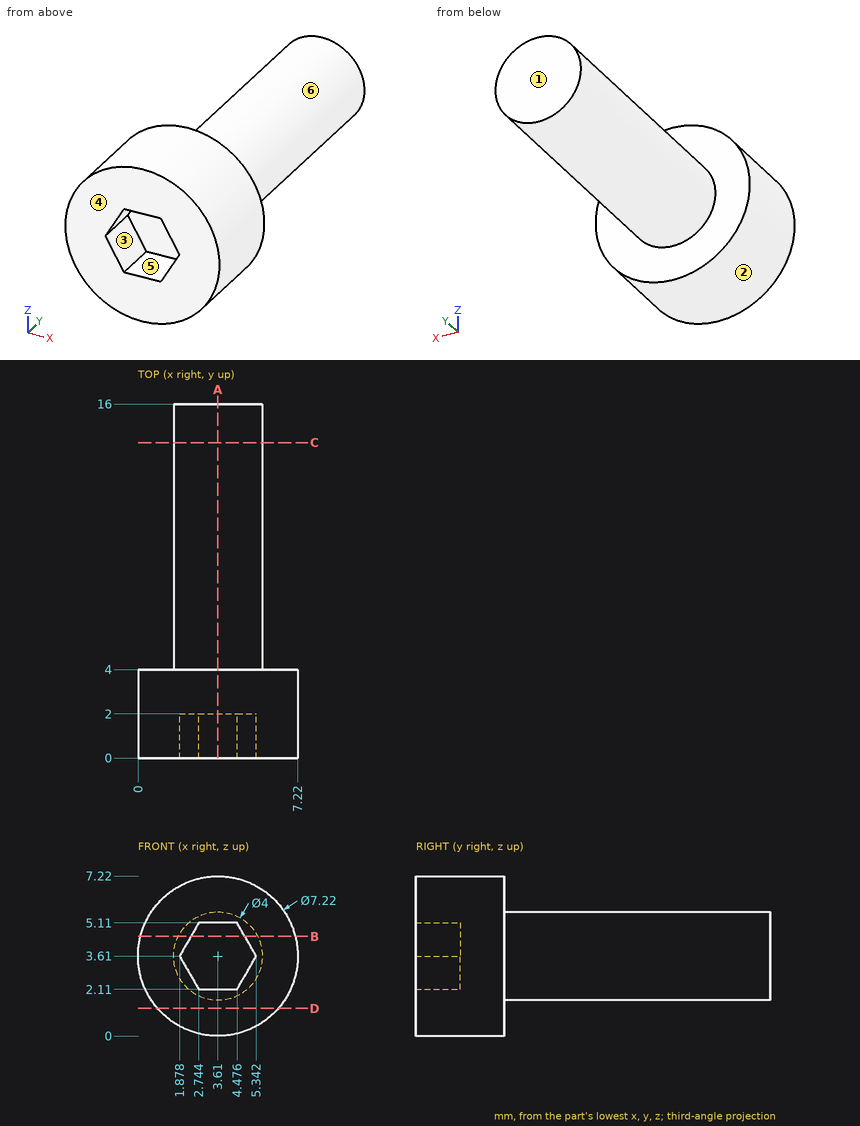
Source: three-view drawing plus pictorial views. Frame: mm from the lowest corner of the part. A direction names the side the tool comes from. Coordinates: 2 decimals unless noted, no trailing zeros. Order: outer loops, then holes, each group sorted by start corner. A loop starts at its lowest first (then second) coordinate and runs counter-clockwise, first axis right, second up. Notation, with made-up numbers: M 27.25,50 L 35.25,50 A30 ccw 35.25,83 Z; hole C 1.5,53.5 d10. An arc over 180 degrees is marked long. Answer in a Markdown table with one row per item.
(1) Section query B-B, the plane z = 4.5. Output: boundary loops of the cut face in (x, y), plus the area to 3 significant figures.
Numbers:
| item | result |
|---|---|
| outline | M 0.11,0 L 2.39,0 L 2.39,2 L 4.83,2 L 4.83,0 L 7.11,0 L 7.11,4 L 5.4,4 L 5.4,16 L 1.82,16 L 1.82,4 L 0.11,4 Z |
| area | 66.1 mm^2 |
(2) Draft query along X for the marked faces 1, 2 and 3. Return one class per face: pulls with the +X half, pulls with the -X half, needs draft (parallel to the pull), parting line crosses it, or undercut.
Numbers:
| item | result |
|---|---|
| face 1 | needs draft |
| face 2 | parting line crosses it |
| face 3 | undercut |
(3) Section query D-D, the plane z = 1.25. Output: boundary loops of the cut face in (x, y).
Numbers:
| item | result |
|---|---|
| outline | M 0.88,0 L 6.34,0 L 6.34,4 L 0.88,4 Z |
(4) Material intervals for line 1 (Y direction, x = 4.5, z = 0.5); line 2 (Y direction, x = 4.5, z = 3.25); line 3 (Z direction, x = 3.5, y = 5), sorted ascending. Write a range as [from, to].
Numbers:
| item | result |
|---|---|
| line 1 | y = [0, 4] |
| line 2 | y = [2, 16] |
| line 3 | z = [1.61, 5.61] |
(5) Section query A-A, the plane x = 3.61. Output: boundary loops of the cut face in (y, z).
Numbers:
| item | result |
|---|---|
| outline | M 0,0 L 4,0 L 4,1.61 L 16,1.61 L 16,5.61 L 4,5.61 L 4,7.22 L 0,7.22 L 0,5.11 L 2,5.11 L 2,2.11 L 0,2.11 Z |
(6) Section query C-C, the plane y = 14.25. Output: boundary loops of the cut face in (x, z).
Numbers:
| item | result |
|---|---|
| outline | C 3.61,3.61 d4 |
(7) Access query for the marked faces 4, 5 and 6. Directions: +Z, -Z, +X, -X, +Y, -Y. A direction counts if a zero-diameter tool reaches every point of the face in a straight line with its end or side. Return the directions, or none.
Numbers:
| item | result |
|---|---|
| face 4 | +Z, -Z, +X, -X, -Y |
| face 5 | -Y |
| face 6 | +Y |
(8) Contact query for flat-ended pins moving along their axis: pin 1 Ø1.5 at (x, y) = (2.5, 13) entering from -Z; pin 2 Ø2 at (y, z) = (7, 2) entering from +X. Output: stop coordinate, or through.
Numbers:
| item | result |
|---|---|
| pin 1 | stops at z = 1.64 |
| pin 2 | stops at x = 5.51 |
